from build123d import *

# Parameters (mm, degrees)
F0_R     = 23.8732414638
F1_DEPTH = 80
F2_R     = 22.8732414638
F3_DEPTH = 80
F5_DEPTH = 80


with BuildPart() as f1:
    # F0 (on Front) → F1 (new body)
    with BuildSketch(Plane.XZ):
        Circle(F0_R)
    extrude(amount=-F1_DEPTH)

    # F2 (on face) → F3 (cut)
    with BuildSketch(Plane.XZ):
        Circle(F2_R)
    extrude(amount=-F3_DEPTH, mode=Mode.SUBTRACT)

    # F4 (on face) → F5 (join)
    with BuildSketch(Plane.XZ):
        with BuildLine():
            ThreePointArc((-16.8741736493, 16.8876855028), (0.0095543232, 23.8732395519), (16.8876855028, 16.8741736493))
            ThreePointArc((16.8876855028, 16.8741736493), (0.0155574816, 38.8732383507), (-16.8741736493, 16.8876855028))
        make_face()
    extrude(amount=-F5_DEPTH)


solid = f1.part
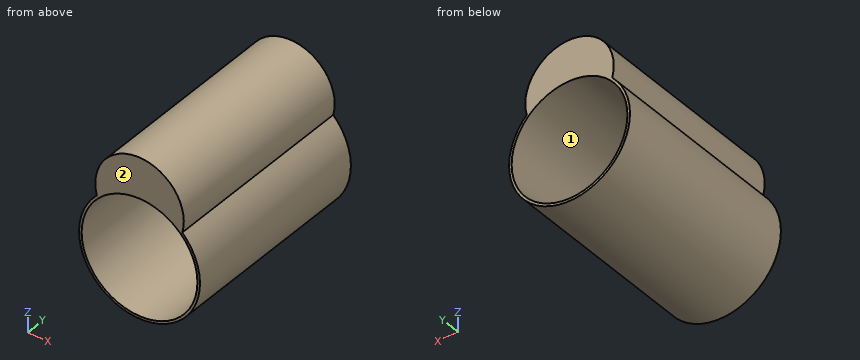
Part model, mm, in its own coordinate system. Face numbers are marked on the shaded views. Give positions to 0.01 mm unless a question says otherwise; leave off trailing zeros. Order: outer loops, then holes, each group sorted by start corner. A loop starts at its lowest first (then second) coordinate and runs counter-clockwise, first axis right, second up. Notation, with made-up numbers: (-9, -35.75) -> (15, -35.75) arc R16 ccw to (15, -5.75) -> close; hole circle Ø10 at (-14, -26.5). An arc over 180 degrees is marked (long way). Use one line per item in the form item = value.
(1) Saw through at C-C (y = 41.5). Write the cut outline in (x, z), then the cut area to 3 significant figures.
Solution:
outline = (-16.87, 16.89) arc R23.87 ccw (long way) to (16.89, 16.87) arc R17.47 ccw (long way) to start; hole circle Ø45.75 at (0, 0)
area = 620 mm²
(2) Saw through at B-B (z = 0). Write the cut outline in (x, y), then the cut area to 3 significant figures.
Solution:
outline = (-23.87, 0) -> (-22.87, 0) -> (-22.87, 80) -> (-23.87, 80) -> close; (22.87, 0) -> (23.87, 0) -> (23.87, 80) -> (22.87, 80) -> close
area = 160 mm²
(3) Flat gauge pins, fed straight in: P1, Ø5, axis at y = 40.5, z = -8.5, coming from the +X side; P2, Ø2, axis at y = 18, z = -2, coming from the -X side; P3, Ø1, axis at x = 3.5, y = 37.5, coming from the -Z side. Where does each tip first touch, or does it go through?
Solution:
P1 = 23.11
P2 = -23.85
P3 = -23.68
(4) Saw through at A-A (x = 0). Write the cut outline in (y, z), then the cut area to 3 significant figures.
Solution:
outline = (0, -23.87) -> (80, -23.87) -> (80, -22.87) -> (0, -22.87) -> close; (0, 22.87) -> (80, 22.87) -> (80, 38.87) -> (0, 38.87) -> close
area = 1,360 mm²
(5) Pull direction Z, two halves, no side cores. Call the marked faces 1 and 2: +Z half, -Z half, draft (parallel to the pull), parting line (faces both ways), or undercut.
Solution:
face_1 = undercut
face_2 = draft
(6) Drill centre lines: line 1 (Z direction, x = 0, y = 38); line 2 (X direction, y = 69, z = -0.5); line 3 (X direction, y = 23, z = -8.5). Where is each one in solid material? Low to high. Write a range as from..to.
Solution:
line_1 = -23.87..-22.87, 22.87..38.87
line_2 = -23.87..-22.87, 22.87..23.87
line_3 = -22.31..-21.24, 21.24..22.31
